```python
from build123d import *

# Parameters (mm, degrees)
SKETCH1_W           = 50
SKETCH1_H           = 44
BOSS_EXTRUDE1_DEPTH = 38.5
M5_TAPPED_HOLE1_D   = 4.2
SKETCH6_R           = 14
CUT_EXTRUDE1_DEPTH  = 45
SKETCH8_R           = 14
SKETCH8_R_2         = 8
BOSS_EXTRUDE2_DEPTH = 18.5


with BuildPart() as part:
    # Sketch1 → Boss-Extrude1 (new body)
    with BuildSketch(Plane.XY):
        Rectangle(SKETCH1_W, SKETCH1_H)
    extrude(amount=BOSS_EXTRUDE1_DEPTH)

    # M5 Tapped Hole1 (through all)
    with Locations(Plane.XY.offset(38.5)):
        with Locations((-18, 17), (18, 17), (18, -17), (-18, -17)):
            Hole(M5_TAPPED_HOLE1_D / 2)

    # Sketch6 → Cut-Extrude1 (cut, through all)
    with BuildSketch(Plane(origin=(0, 22, 0), x_dir=(1, 0, 0), z_dir=(0, 1, 0))):
        with Locations((0, -19.5)):
            Circle(SKETCH6_R)
        Polygon((-25, -10.5), (-14.5, 0), (-25, 0), align=None)
        Polygon((25, -10.5), (14.5, 0), (25, 0), align=None)
    extrude(amount=-CUT_EXTRUDE1_DEPTH, mode=Mode.SUBTRACT)

    # Sketch8 → Boss-Extrude2 (add, symmetric)
    with BuildSketch(Plane(origin=(0, 0, 0), x_dir=(-1, 0, 0), z_dir=(0, -1, 0))):
        with Locations((0, -19.5)):
            Circle(SKETCH8_R)
        with Locations((0, -19.5)):
            Circle(SKETCH8_R_2, mode=Mode.SUBTRACT)
    extrude(amount=BOSS_EXTRUDE2_DEPTH, both=True)


solid = part.part
```
Model file for the job. Use its own axes, mm. A direction names the side the tool comes from. Coordinates: 2 decimals unless noted, no trailing zeros. Write each loop counter-clockwise with the first axis right and the second up, starting at its lowest first coordinate (ties: lowest second). Pieces come first, ordered by that corner, then holes. Notation, with made-up numbers: (-11, -25) - (13, -25) arc R5 ccw to (13, -18) - close; hole circle Ø4 at (-15, 46.5). An arc over 180 degrees is marked (long way). One line per item, written item: value. Start each with the question number.
1. Slice it at C-C (x = 0). Write the cut outline in (y, z), plus the area to 3 significant figures.
2. Slice it at B-B (z = 19.5). Write the cut outline in (x, y), plus the area to 3 significant figures.
3. Probe line 1 (Y direction, x = -18, z = 31); line 2 (X direction, y = -17, z = 30); line 3 (Y direction, x = -17, z = 10). List the from-to ranges inside material, lowest first. Write a range as from..to.
4. Tool access for faces 1 (the cylindrical face through (-3.03, 20.27, 33.17)), 2 (the cylindrical face through (-3.03, -20.23, 33.17)), 3 (the flat face through (19.8, 0.3, 5.3)): list every direction of +Z, -Z, +X, -X, +Y, -Y with a clear straight run to the whole face (end or side of a thin tool).
5. Flat gauge pins, fed straight in: pin 1 (17 mm diameter, centred on x = 0, z = 19.5, fed in from +Y); pin 2 (1 mm diameter, centred on y = -1, z = 4.5, fed in from +X). Where does each tip first touch, or does it go through?
6. Slice it at A-A (y = 17). Write the cut outline in (x, z), plus the area to 3 significant figures.
7. Slice it at D-D (x = 18). Write the cut outline in (y, z).
8. Mould opens along X. For faces 4 (the flat face through (25, 0, 24)), 5 (the flat face through (-6, -18.5, 26)), 6 (the flat face through (-19.8, 0.3, 5.3)), 7 (the flat face through (11, 22, 10)) say: released by +X, released by -X, zero draft, split by the parting line, or undercut.
Answers below:
1. outline: (-22, 0) - (22, 0) - (22, 5.5) - (18.5, 5.5) - (18.5, 11.5) - (-18.5, 11.5) - (-18.5, 5.5) - (-22, 5.5) - close; (-22, 33.5) - (-18.5, 33.5) - (-18.5, 27.5) - (18.5, 27.5) - (18.5, 33.5) - (22, 33.5) - (22, 38.5) - (-22, 38.5) - close
1. area: 906 mm^2
2. outline: (-25, -22) - (-14, -22) - (-14, -18.5) - (-8, -18.5) - (-8, 18.5) - (-14, 18.5) - (-14, 22) - (-25, 22) - close; (8, -18.5) - (14, -18.5) - (14, -22) - (25, -22) - (25, 22) - (14, 22) - (14, 18.5) - (8, 18.5) - close; hole circle Ø4.2 at (-18, -17); hole circle Ø4.2 at (-18, 17); hole circle Ø4.2 at (18, -17); hole circle Ø4.2 at (18, 17)
2. area: 1,360 mm^2
3. line 1: y = -22..-19.1, -14.9..14.9, 19.1..22
3. line 2: x = -25..-20.1, -15.9..15.9, 20.1..25
3. line 3: y = -22..-18.85, -15.15..15.15, 18.85..22
4. face 1: +Y
4. face 2: -Y
4. face 3: -Z, +X, +Y, -Y
5. pin 1: stops at y = 18.5
5. pin 2: stops at x = 19.5
6. outline: (-25, 10.5) - (-20.1, 5.6) - (-20.1, 38.5) - (-25, 38.5) - close; (-15.9, 1.4) - (-14.5, 0) - (14.5, 0) - (15.9, 1.4) - (15.9, 38.5) - (-15.9, 38.5) - close; (20.1, 5.6) - (25, 10.5) - (25, 38.5) - (20.1, 38.5) - close; hole circle Ø16 at (0, 19.5)
6. area: 1,320 mm^2
7. outline: (-22, 3.5) - (-19.1, 3.5) - (-19.1, 38.5) - (-22, 38.5) - close; (-14.9, 3.5) - (14.9, 3.5) - (14.9, 38.5) - (-14.9, 38.5) - close; (19.1, 3.5) - (22, 3.5) - (22, 38.5) - (19.1, 38.5) - close
8. face 4: released by +X
8. face 5: undercut
8. face 6: released by -X
8. face 7: zero draft
